```python
from build123d import *

# Parameters (mm, degrees)
F0_W     = 18.923
F0_H     = 6.985
F1_DEPTH = 22.86
F3_DEPTH = 0.635
F5_DEPTH = 5.08
F4_W     = 1.143
F4_H     = 3.175
F6_DEPTH = 6.985
F7_W     = 1.143
F7_H     = 2.54
F8_DEPTH = 12.7


# Not quite as in the source:
# - a feature names something its author has since deleted; it is built from what else it names


with BuildPart() as f1:
    # F0 (on Front) → F1 (new body)
    with BuildSketch(Plane.XZ):
        with Locations((0, -0.3175)):
            Rectangle(F0_W, F0_H)
    extrude(amount=F1_DEPTH)

    # F2 (on face) → F3 (join)
    with BuildSketch(Plane.XZ.offset(22.86)):
        Polygon((9.9764279214, 4.318), (-9.9695, 4.318), (-9.9695, -3.81), (-9.4615, -3.81), (-9.4615, 3.175), (9.4615, 3.175), (9.4615, -3.81), (9.9764279214, -3.81), align=None)
    extrude(amount=-F3_DEPTH)

    # F4 (on face) → F5 (cut)
    with BuildSketch(Plane.XY.offset(3.175)):
        with BuildLine():
            ThreePointArc((5.9100590949, -9.232738686), (5.9100590949, -8.724738686), (5.4701181898, -8.470738686))
            Line((5.4701181898, -8.470738686), (-5.4701181898, -8.470738686))
            ThreePointArc((-5.4701181898, -8.470738686), (-5.9100590949, -8.724738686), (-5.9100590949, -9.232738686))
            Line((-5.9100590949, -9.232738686), (-0.4399409051, -18.707261314))
            ThreePointArc((-0.4399409051, -18.707261314), (0, -18.961261314), (0.4399409051, -18.707261314))
            Line((0.4399409051, -18.707261314), (5.9100590949, -9.232738686))
        make_face()
    extrude(amount=-F5_DEPTH, mode=Mode.SUBTRACT)

    # F4 (on face) → F6 (join, through all)
    with BuildSketch(Plane.XY.offset(3.175)):
        with Locations((-10.033, -1.5875)):
            Rectangle(F4_W, F4_H)
        with Locations((10.033, -1.5875)):
            Rectangle(F4_W, F4_H)
    extrude(amount=-F6_DEPTH)

    # F7 (on face) → F8 (cut)
    with BuildSketch(Plane.XZ):
        with Locations((10.033, 0)):
            Rectangle(F7_W, F7_H)
        with Locations((-10.033, 0)):
            Rectangle(F7_W, F7_H)
    extrude(amount=F8_DEPTH, mode=Mode.SUBTRACT)


solid = f1.part
```
Part model, mm, in its own coordinate system. A direction names the side the tool comes from. Round coordinates to 2 decimals unless told otherwise and drop trailing zeros. Loops run counter-clockwise (first coordinate to the right, second up) from the corner with the lowest first, then second, coordinate; pieces in that order, holes last. Notation, with made-up numbers: (72.25, -33) -> (96.25, -33) arc R33 ccw to (96.25, -1) -> close; hole circle Ø2 at (88, 59.5). An arc over 180 degrees is marked (long way). Use CSV: the item, a comma, the result in double quotes. Start each with the question number.
1) Cut at A-A, the plane z = -1. Write the cut outline in (x, y) (1 decimal), plus the area to 3 significant figures.
2) Cut at B-B, the plane y = -2. Write the cut outline in (x, z) (1 decimal).
3) Drop flat-ended pins along their axis: P1, Ø1, axis at x = 3.5, y = -3, coming from the +Z side (3 decimals); P2, Ø2, axis at x = -1.5, y = -12.5, coming from the +Z side (3 decimals); P3, Ø0.5, axis at y = -22.5, z = 2, coming from the -X side. Give the stop position or say it passes through.
4) Cut at C-C, the plane x = 8.75. Write the cut outline in (y, z) (3 decimals).
5) Which spindle directions (+Z, -Z, +X, -X, +Y, -Y) get a long thin tool onto all of the face, cutting with end or side? Do faces 4 (the flat face through (10, -3.175, -3)), 5 (the flat face through (10, -2, 1.27)), 6 (the flat face through (-10, -3.175, -3)), 7 (the flat face through (-3.213, -13.904, 0.671)). Say none if no direction does.
6) Pull direction Z, two halves, no side cores. Call faces 1 (the flat face through (-10, -2, -1.27)), 2 (the flat face through (0, -22.86, 0)), 3 (the flat face through (0, -11, -3.81)): +Z half, -Z half, draft (parallel to the pull), parting line (faces both ways), or undercut.
7) Wall check: L1, parallel to X at y = -8.25, z = 3; L2, parallel to Z at x = 6.5, y = -7.25 (3 decimals); L3, parallel to Y at x = -2, z = 3.25 (3 decimals). Give the ranges that are in metal, low to high. Write a range as [from, to].
8) Cut at D-D, the plane z = 2.5. Write the cut outline in (x, y) (1 decimal), plus the area to 3 significant figures.
Determined:
1,outline,"(-10, -22.9) -> (10, -22.9) -> (10, -22.2) -> (9.5, -22.2) -> (9.5, 0) -> (-9.5, 0) -> (-9.5, -22.2) -> (-10, -22.2) -> close; hole (-5.9, -9.2) -> (-0.4, -18.7) arc R0.5 ccw to (0.4, -18.7) -> (5.9, -9.2) arc R0.5 ccw to (5.5, -8.5) -> (-5.5, -8.5) arc R0.5 ccw to start"
1,area,"364 mm2"
2,outline,"(-10.6, -3.8) -> (10.6, -3.8) -> (10.6, -1.3) -> (9.5, -1.3) -> (9.5, 1.3) -> (10.6, 1.3) -> (10.6, 3.2) -> (-10.6, 3.2) -> (-10.6, 1.3) -> (-9.5, 1.3) -> (-9.5, -1.3) -> (-10.6, -1.3) -> close"
3,P1,"stops at z = 3.175"
3,P2,"stops at z = -1.905"
3,P3,"stops at x = -9.97"
4,outline,"(-22.86, -3.81) -> (0, -3.81) -> (0, 3.175) -> (-22.225, 3.175) -> (-22.225, 4.318) -> (-22.86, 4.318) -> close"
5,face 4,"+Z, -Z, +X"
5,face 5,"+X, +Y"
5,face 6,"+Z, -Z, -X"
5,face 7,"+Z"
6,face 1,"undercut"
6,face 2,"draft"
6,face 3,"-Z half"
7,L1,"x = [-9.46, 9.46]"
7,L2,"z = [-3.81, 3.175]"
7,L3,"y = [-22.86, -22.225]"
8,outline,"(-10.6, -3.2) -> (-9.5, -3.2) -> (-9.5, -22.2) -> (-10, -22.2) -> (-10, -22.9) -> (10, -22.9) -> (10, -22.2) -> (9.5, -22.2) -> (9.5, -3.2) -> (10.6, -3.2) -> (10.6, 0) -> (-10.6, 0) -> close; hole (-5.9, -9.2) -> (-0.4, -18.7) arc R0.5 ccw to (0.4, -18.7) -> (5.9, -9.2) arc R0.5 ccw to (5.5, -8.5) -> (-5.5, -8.5) arc R0.5 ccw to start"
8,area,"371 mm2"
